```python
from build123d import *

# Parameters (mm, degrees)
SKETCH1_R           = 4
SKETCH1_R_2         = 3
BOSS_EXTRUDE1_DEPTH = 10


with BuildPart() as part:
    # Sketch1 → Boss-Extrude1 (new body)
    with BuildSketch(Plane(origin=(0, 0, 0), x_dir=(0, 0, -1), z_dir=(1, 0, 0))):
        with BuildLine():
            Line((-10, -7.745966692), (-10, -14))
            Line((-10, -14), (10, -14))
            Line((10, -14), (10, -7.745966692))
            Line((10, -7.745966692), (17.5, -5.809475019))
            ThreePointArc((17.5, -5.809475019), (22, 0), (17.5, 5.809475019))
            Line((17.5, 5.809475019), (2.5, 9.682458366))
            ThreePointArc((2.5, 9.682458366), (0, 10), (-2.5, 9.682458366))
            Line((-2.5, 9.682458366), (-17.5, 5.809475019))
            ThreePointArc((-17.5, 5.809475019), (-22, 0), (-17.5, -5.809475019))
            Line((-17.5, -5.809475019), (-10, -7.745966692))
        make_face()
        Circle(SKETCH1_R, mode=Mode.SUBTRACT)
        with Locations((16, 0)):
            Circle(SKETCH1_R_2, mode=Mode.SUBTRACT)
        with Locations((-16, 0)):
            Circle(SKETCH1_R_2, mode=Mode.SUBTRACT)
    extrude(amount=BOSS_EXTRUDE1_DEPTH)


solid = part.part
```
The model under review builds one solid part; all positions refer to its coordinate system, in mm. A direction names the side the tool comes from. Give positions to 0.01 mm unless a question says otherwise; leave off trailing zeros. Write each loop counter-clockwise with the first axis right and the second up, starting at its lowest first coordinate (ties: lowest second). Pieces come first, ordered by that corner, then holes. Notation, with made-up numbers: (79.5, 38) - (121.5, 38) arc R19 cw to (121.5, 61) - close; hole circle Ø9 at (-18, 10). An arc over 180 degrees is marked (long way). Answer in a Markdown table with one row per item. Add a question column.
1. Wall thickness on line 1 along Z through (x, y) = (6.75, -0.75); line 2 along Z through (x, y) = (4, 1); line 3 along Y through (x, z) = (3, 0): over which ranges is each line inside the solid? List them lowest first. Write a range as [from, to].
2. Insertion check: P1, Ø3, axis at x = 3, y = -5, coming from the -Z side; P2, Ø3, axis at x = 6.5, y = -12.5, coming from the +Z side; P3, Ø1.5, axis at x = 4.5, y = 2.5, coming from the -Z side. Each pin has a flat end and moves straight along its axis. Give the tip position at first contact, or say it passes through.
3. Draft analysis for pull direction Y (two halves, no side actions). For faces 4 (the cylindrical face through (5, 0, 19)), 5 (the flat face through (10, -4.5, 0.3)), 6 (the flat face through (4.93, 7.72, -10.1)), state which applies: +Y half, -Y half, draft (parallel to the pull), parting line (faces both ways), or undercut.
4. We need section C-C on x = 6.75. Write out the cut boundary in (y, z), then the cut area to 3 significant figures.
5. Tool access review of faces 1 (the cylindrical face through (5, 0, -13)), 2 (the flat face through (5, -11, 10)), 3 (the flat face through (5, -11, -10)): name each direction out of +Z, -Z, +X, -X, +Y, -Y from which nothing blocks a thin tool from reaching the whole face with its end or side.
6. We need section A-A on y = 0. Write out the cut boundary in (x, z).
7. We need section D-D on y = -3.5. Write out the cut boundary in (x, z), then the cut area to 3 significant figures.
8. We need section B-B on z = 0. Write out the cut boundary in (x, y), then the cut area to 3 significant figures.
Ans:
| question | item | result |
|---|---|---|
| 1 | line 1 | z = [-21.95, -18.9], [-13.1, -3.93], [3.93, 13.1], [18.9, 21.95] |
| 1 | line 2 | z = [-21.92, -18.83], [-13.17, -3.87], [3.87, 13.17], [18.83, 21.92] |
| 1 | line 3 | y = [-14, -4], [4, 10] |
| 2 | P1 | stops at z = -20.87 |
| 2 | P2 | stops at z = 10 |
| 2 | P3 | stops at z = -21.74 |
| 3 | face 4 | undercut |
| 3 | face 5 | draft |
| 3 | face 6 | +Y half |
| 4 | outline | (-14, -10) - (-7.75, -10) - (-5.81, -17.5) arc R6 ccw to (5.81, -17.5) - (9.68, -2.5) arc R10 ccw to (9.68, 2.5) - (5.81, 17.5) arc R6 ccw to (-5.81, 17.5) - (-7.75, 10) - (-14, 10) - close; hole circle Ø8 at (0, 0); hole circle Ø6 at (0, -16); hole circle Ø6 at (0, 16) |
| 4 | area | 634 mm^2 |
| 5 | face 1 | +X, -X |
| 5 | face 2 | +Z, +X, -X, -Y |
| 5 | face 3 | -Z, +X, -X, -Y |
| 6 | outline | (0, -22) - (10, -22) - (10, -19) - (0, -19) - close; (0, -13) - (10, -13) - (10, -4) - (0, -4) - close; (0, 4) - (10, 4) - (10, 13) - (0, 13) - close; (0, 19) - (10, 19) - (10, 22) - (0, 22) - close |
| 7 | outline | (0, -20.87) - (10, -20.87) - (10, -1.94) - (0, -1.94) - close; (0, 1.94) - (10, 1.94) - (10, 20.87) - (0, 20.87) - close |
| 7 | area | 379 mm^2 |
| 8 | outline | (0, -14) - (10, -14) - (10, -4) - (0, -4) - close; (0, 4) - (10, 4) - (10, 10) - (0, 10) - close |
| 8 | area | 160 mm^2 |
